Autodesk Inventor part; units mm, degrees
ref_plane "Work Plane1" through (0, -9.375, 25) normal (0, -1, 0) x (1, 0, 0)
ref_plane "YZ Plane" through (0, 0, 0) normal (1, 0, 0) x (0, 1, 0)
ref_plane "XZ Plane" through (0, 0, 0) normal (0, 1, 0) x (-1, 0, 0)
sketch "Sketch1" plane through (0, 0, 0) normal (0, 0, 1) x (1, 0, 0)
  circle A0 centre (0, 0) radius 9.375
  circle A1 centre (0, 0) radius 2.5
  dimension "d0" = 18.75
  dimension "d1" = 5
extrude "Extrusion1" add sketch "Sketch1" along normal blind 25
sketch "Point of Tangency + Nut" plane through (0, 0, 25) normal (0, 0, 1) x (1, 0, 0)
  circle A0 centre (0, 0) radius 9.375
  line L0 (0, -9.375) -> (0, -2.5) construction
  circle A1 centre (0, 0) radius 2.5 construction
  line L1 (2.75, -7.4375) -> (-2.75, -7.4375)
  line L2 (-2.75, -7.4375) -> (-2.75, -4.4375)
  line L3 (-2.75, -4.4375) -> (2.75, -4.4375)
  line L4 (2.75, -4.4375) -> (2.75, -7.4375)
  line L5 (2.75, -7.4375) -> (-2.75, -4.4375) construction
  line L6 (-2.75, -7.4375) -> (2.75, -4.4375) construction
  point P0 (0, -5.9375)
  dimension "d8" = 5.5
  dimension "d9" = 3
ref_plane "Work Plane1" through (0, -9.375, 25) normal (0, -1, 0) x (1, 0, 0)
sketch "Sketch3" plane through (0, -9.375, 25) normal (0, -1, 0) x (1, 0, 0)
  line L0 (9.375, 0) -> (-9.375, 0) construction
  line L1 (0, 0) -> (0, -6) construction
  circle A0 centre (0, -6) radius 1.5
  point P0 (0, -25)
  dimension "d4" = 6
  dimension "d5" = 3
extrude "LocBolt" cut sketch "Sketch3" against normal blind 8
extrude "LocNut Gap" cut sketch "Point of Tangency + Nut" against normal blind 9.5 contours L1 L2 L3 L4
properties part number "MotorTripodCoupler"
The listing builds one solid part. Answer for the finished solid, in the listing's coordinates (mm). A direction names the side the tool comes from. Give positions to 0.01 mm unless a question says otherwise; leave off trailing zeros. Loops run counter-clockwise (first coordinate to the right, second up) from the corner with the lowest first, then second, coordinate; pieces in that order, holes last. Notation, with made-up numbers: (-13, -24.5) - (43, -24.5) arc R18 cw to (43, 8.5) - close; hole circle Ø9 at (46, 29). An arc over 180 degrees is marked (long way). Answer as CSV lines item,"result". Start each with the question number.
Item 1: A cutting plane is placed at C-C on z = 3. Determine the outline of the cut face in (x, y) (3 decimals), then the cut area to 3 significant figures.
Item 2: Each of these flat-tipped pins is pushed along its axis until it touches: pin 1 (2.5 mm diameter, centred on x = 0, z = 19, fed in from -Y); pin 2 (2.5 mm diameter, centred on y = -5.5, z = 18, fed in from -X); pin 3 (4.5 mm diameter, centred on x = 0.5, z = 21, fed in from +Y) (3 decimals); pin 4 (1 mm diameter, centred on x = -4, z = 12.5, fed in from +Y). Where does it stop, or does it pass through?
Item 3: Find the intervals of material crossed by line 1 (Y direction, x = 0, z = 16.75) (1 decimal); line 2 (Z direction, x = 0, y = -8.6); line 3 (Y direction, x = 1.75, z = 17.25), in increasing order. Write a range as from..to.
Item 4: For faces 5 (the face through (-2.75, -6, 20)), 6 (the face through (-0.54, 2.44, 12.32)), 7 (the face through (1.43, -3.24, 19.45)), determine the directions among +Z, -Z, +X, -X, +Y, -Y from which every point of the face is accessible in a straight line to the end or side of a thin tool.
Item 5: The mould has two halves that part along X. Classify faces 1 (the face through (2, 2, 25)), 2 (the face through (0, -4.438, 21)), 3 (the face through (-1.5, -8.42, 19.07)), 4 (the face through (-1.22, -9.295, 12.325)): +X half, -X half, draft (parallel to the pull), parting line (faces both ways), or undercut.
Item 6: A cutting plane is placed at B-B on x = 0. Determine the outline of the cut face in (y, z) (1 decimal), then the cut area to 3 significant figures.
Item 7: A cutting plane is placed at A-A on y = 0. Determine the outline of the cut face in (x, z) (3 decimals), then the cut area to 3 significant figures.
Found:
1,outline,"circle Ø18.75 at (0, 0); hole circle Ø5 at (0, 0)"
1,area,"256 mm^2"
2,pin 1,"stops at y = 2.17"
2,pin 2,"stops at x = -8.36"
2,pin 3,"stops at y = 9.375"
2,pin 4,"stops at y = 8.7"
3,line 1,"y = -9.4..-7.4, -4.4..-2.5, 2.5..9.4"
3,line 2,"z = 0..17.5, 20.5..25"
3,line 3,"y = -9.21..-7.44, -4.44..-1.79, 1.79..9.21"
4,face 5,"+Z"
4,face 6,"+Z, -Z"
4,face 7,"-Y"
5,face 1,"draft"
5,face 2,"undercut"
5,face 3,"undercut"
5,face 4,"parting line"
6,outline,"(-9.4, 0) - (-2.5, 0) - (-2.5, 17.5) - (-4.4, 17.5) - (-4.4, 15.5) - (-7.4, 15.5) - (-7.4, 17.5) - (-9.4, 17.5) - close; (-9.4, 20.5) - (-7.4, 20.5) - (-7.4, 25) - (-9.4, 25) - close; (-4.4, 20.5) - (-2.5, 20.5) - (-2.5, 25) - (-4.4, 25) - close; (2.5, 0) - (9.4, 0) - (9.4, 25) - (2.5, 25) - close"
6,area,"304 mm^2"
7,outline,"(-9.375, 0) - (-2.5, 0) - (-2.5, 25) - (-9.375, 25) - close; (2.5, 0) - (9.375, 0) - (9.375, 25) - (2.5, 25) - close"
7,area,"344 mm^2"
